from build123d import *

# Parameters (mm, degrees)
ESQUISSE1_W                   = 12.5
ESQUISSE1_H                   = 2
ESQUISSE2_R                   = 6
BOSS_EXTRU_1_DEPTH            = 15
DIAM_TRE_DU_PER_AGE_3_0_3_1_D = 3
D_GAGEMENT_M21_D              = 2.459
D_GAGEMENT_M21_DEPTH          = 17


with BuildPart() as part:
    # Esquisse1 → Révolution1 (revolve)
    with BuildSketch(Plane(origin=(0, 152.70275651, 0), x_dir=(1, 0, 0), z_dir=(0, 1, 0))):
        with Locations((177.420752313, -1)):
            Rectangle(ESQUISSE1_W, ESQUISSE1_H)
    revolve(axis=Axis((171.170752313, 152.70275651, 0), (0, 0, 1)))

    # Esquisse2 → Boss.-Extru.1 (add)
    with BuildSketch(Plane.XY.offset(2)):
        with Locations((171.170752313, 152.70275651)):
            Circle(ESQUISSE2_R)
    extrude(amount=BOSS_EXTRU_1_DEPTH)

    # Diamètre du perçage Ø3.0 (3)1 (through all)
    with Locations(Plane(origin=(0, 0, 0), x_dir=(-1, 0, 0), z_dir=(0, 0, -1))):
        with Locations((-171.170752313, 152.70275651)):
            Hole(DIAM_TRE_DU_PER_AGE_3_0_3_1_D / 2)

    # Dégagement M21
    with Locations(Plane(origin=(0, 0, 0), x_dir=(-1, 0, 0), z_dir=(0, 0, -1))):
        with Locations((-179.170752313, 152.70275651), (-163.170752313, 152.70275651), (-171.170752313, 162.20275651), (-171.170752313, 143.20275651)):
            Hole(D_GAGEMENT_M21_D / 2, depth=D_GAGEMENT_M21_DEPTH)


solid = part.part
Geometry check sheet. Reference: the model listing, model coordinates, mm. A direction names the side the tool comes from. Coordinates: 2 decimals unless noted, no trailing zeros. Order: outer loops, then holes, each group sorted by start corner. A loop starts at its lowest first (then second) coordinate and runs counter-clockwise, first axis right, second up. Notation, with made-up numbers: (17.5, -18) - (33.5, -18) arc R17 cw to (33.5, 3) - close; hole circle Ø3 at (10.5, 64). An arc over 180 degrees is marked (long way). One line per item, written item: value.
(1) Access from +Z, -Z, +X, -X, +Y, -Y to the whole of each face (thin tool, end or side, straight path). Record for faces 4 (the face through (172.343, 143.572, 1.014)), 5 (the face through (174, 147, 2)).
Data:
face 4: +Z, -Z
face 5: +Z
(2) Sectioned sample at B-B (y = 142.75). Enter the section's corners in (x, z), and give its area (3 significant figures).
Data:
outline: (163.61, 0) - (170.03, 0) - (170.03, 2) - (163.61, 2) - close; (172.31, 0) - (178.73, 0) - (178.73, 2) - (172.31, 2) - close
area: 25.7 mm^2
(3) Sectioned sample at A-A (x = 170.5). Enter the section's corners in (y, z), and give its area (3 significant figures).
Data:
outline: (140.22, 0) - (142.17, 0) - (142.17, 2) - (140.22, 2) - close; (144.23, 0) - (151.36, 0) - (151.36, 17) - (146.74, 17) - (146.74, 2) - (144.23, 2) - close; (154.04, 0) - (161.17, 0) - (161.17, 2) - (158.67, 2) - (158.67, 17) - (154.04, 17) - close; (163.23, 0) - (165.18, 0) - (165.18, 2) - (163.23, 2) - close
area: 175 mm^2
(4) Sectioned sample at C-C (z = 1). Enter the section's corners in (x, y).
Data:
outline: circle Ø25 at (171.17, 152.7); hole circle Ø2.46 at (163.17, 152.7); hole circle Ø3 at (171.17, 152.7); hole circle Ø2.46 at (171.17, 143.2); hole circle Ø2.46 at (171.17, 162.2); hole circle Ø2.46 at (179.17, 152.7)
(5) Thickness scan on probe 1 along Z at (x, y) = (164.75, 145.75); probe 2 along X at (y, z) = (152.5, 2.25); probe 3 along X at (y, z) = (154, 14.5). Record the ranges inside material, lowest first. Write a range as from..to.
Data:
probe 1: z = 0..2
probe 2: x = 165.17..169.68, 172.66..177.17
probe 3: x = 165.31..170.42, 171.92..177.03
(6) Release check for a two-part mould opening along X. For faces 1 (the face through (162.2, 151.95, 1.01)), 2 (the face through (171, 150, 0)), 3 (the face through (158.683, 153.252, 0.986)) record: +X half, -X half, draft (parallel to the pull), parting line (faces both ways), or undercut.
Data:
face 1: undercut
face 2: draft
face 3: parting line
(7) Sectioned sample at D-D (x = 163.5). Enter the section's corners in (y, z).
Data:
outline: (142.83, 0) - (151.52, 0) - (151.52, 2) - (142.83, 2) - close; (153.89, 0) - (162.57, 0) - (162.57, 2) - (153.89, 2) - close
(8) Depth check by flat-ended pin: pin 1 Ø5 at (x, z) = (165.5, 5.5) entering from +Y; pin 2 Ø8 at (x, z) = (177.5, 3.5) entering from +Y; pin 3 Ø10 at (y, z) = (160, 15) entering from -X. Enter the tip coordinate at first touch or a pass-through.
Data:
pin 1: stops at y = 157.8
pin 2: stops at y = 164.92
pin 3: stops at x = 165.63
